Geometry: final body of the model. Coordinates: model frame, mm. Round coordinates to 2 decimals unless told otherwise and drop trailing zeros. Order: outer loops, then holes, each group sorted by start corner. A loop starts at its lowest first (then second) coordinate and runs counter-clockwise, first axis right, second up. Notation, with made-up numbers: M 47.25,47 L 62.25,47 A26 ccw 62.25,70 Z; hole C -7.5,11.5 d8. An arc over 180 degrees is marked long. Return JSON: item names as keys, results as strings. Group by question number.
Q1. Ray query, probe 1 along Y at (x, z) = (0, 1.3); probe 2 along Y at (x, z) = (-1.5, 0.9). Return the intervals inside material, ascending.
Q2. Contact query for a flat-ended pin moving along its axis: pin 1 (4.5 mm diameter, centred on x = 0, y = 0, fed in from -Z). Output: stop coordinate, or through.
Q3. Mould query, pull axis X, two halves, no side actions, for faces 1 (the face through (0, -3.75, 1)), 2 (the face through (3.75, 0, 1)), 3 (the face through (0, -2, 1)). Classes: released by +X, released by -X, zero draft, split by the parting line, or undercut.
Q4. Cut plane A-A on z = 1.4. Output: boundary loops of the cut face in (x, y).
```python
from build123d import *

# Parameters (mm, degrees)
SKETCH001_W     = 10
SKETCH001_H     = 10
SKETCH001_W_2   = 7.5
SKETCH001_H_2   = 7.5
POCKET_DEPTH    = 5
SKETCH002_R     = 2
POCKET001_DEPTH = 5


with BuildPart() as part:
    # Sketch → Revolution (revolve)
    with BuildSketch(Plane.XZ):
        with BuildLine():
            add(Edge.make_bspline(
                [(0, 2), (4.7, 1.7), (4.9, 1.5)],
                knots=[0, 0, 0, 1, 1, 1], degree=2))
            Line((4.9, 1.5), (4.9, 0))
            add(Edge.make_bspline(
                [(0, 0.5), (3.9, 0.3), (4.9, 0)],
                knots=[0, 0, 0, 1, 1, 1], degree=2))
            Line((0, 0.5), (0, 2))
        make_face()
    revolve(axis=Axis((0, 0, 0), (0, 0, 1)))

    # Sketch001 → Pocket (cut)
    with BuildSketch(Plane.XY):
        Rectangle(SKETCH001_W, SKETCH001_H)
        Rectangle(SKETCH001_W_2, SKETCH001_H_2, mode=Mode.SUBTRACT)
    extrude(amount=POCKET_DEPTH, mode=Mode.SUBTRACT)

    # Sketch002 → Pocket001 (cut)
    with BuildSketch(Plane.XY):
        Circle(SKETCH002_R)
    extrude(amount=POCKET001_DEPTH, mode=Mode.SUBTRACT)


solid = part.part
```
Result sheet:
{
 "1": {"probe 1": "y = -3.75 to -2, 2 to 3.75", "probe 2": "y = -3.75 to -1.32, 1.32 to 3.75"},
 "2": {"pin 1": "stops at z = 0.36"},
 "3": {"face 1": "zero draft", "face 2": "released by +X", "face 3": "undercut"},
 "4": {"outline": "M -3.75,-3.15 A4.9 ccw -3.15,-3.75 L 3.15,-3.75 A4.9 ccw 3.75,-3.15 L 3.75,3.15 A4.9 ccw 3.15,3.75 L -3.15,3.75 A4.9 ccw -3.75,3.15 Z; hole C 0,0 d4"}
}
